Part model, mm, in its own coordinate system. A direction names the side the tool comes from. Give positions to 0.01 mm unless a question says otherwise; leave off trailing zeros. Write each loop counter-clockwise with the first axis right and the second up, starting at its lowest first coordinate (ties: lowest second). Pieces come first, ordered by that corner, then holes. Notation, with made-up numbers: M 62.5,-9.75 L 87.5,-9.75 A36 ccw 87.5,26.25 Z; hole C 64.5,41 d10. An arc over 180 degrees is marked long. Use a Markdown table: item, result. Add a question column.
from build123d import *

# Parameters (mm, degrees)
BOSS_EXTRUDE2_DEPTH = 34.29
CHAMFER1_SIZE       = 2.54
CHAMFER2_SIZE       = 2.54


with BuildPart() as part:
    # Sketch2 → Boss-Extrude2 (new body)
    with BuildSketch(Plane.XY):
        with BuildLine():
            Line((-29.230640855, 30.0736), (29.230640855, 30.0736))
            ThreePointArc((29.230640855, 30.0736), (33.347275907, 29.151687047), (36.677508311, 26.562061635))
            Line((36.677508311, 26.562061635), (49.972274675, 10.43878478))
            ThreePointArc((49.972274675, 10.43878478), (51.110407437, -8.880095747), (33.055391111, -15.846506335))
            Line((33.055391111, -15.846506335), (9.525, -9.525))
            Line((9.525, -9.525), (9.525, -4.1275))
            ThreePointArc((9.525, -4.1275), (10.268948776, -2.331448776), (12.065, -1.5875))
            Line((12.065, -1.5875), (28.178527264, -1.5875))
            ThreePointArc((28.178527264, -1.5875), (46.5836, 0), (28.178527264, 1.5875))
            Line((28.178527264, 1.5875), (-28.178527264, 1.5875))
            ThreePointArc((-28.178527264, 1.5875), (-46.5836, 0), (-28.178527264, -1.5875))
            Line((-28.178527264, -1.5875), (-12.065, -1.5875))
            ThreePointArc((-12.065, -1.5875), (-10.268948776, -2.331448776), (-9.525, -4.1275))
            Line((-9.525, -4.1275), (-9.525, -9.525))
            Line((-9.525, -9.525), (-33.055391111, -15.846506335))
            ThreePointArc((-33.055391111, -15.846506335), (-51.110407437, -8.880095747), (-49.972274675, 10.43878478))
            Line((-49.972274675, 10.43878478), (-36.677508311, 26.562061635))
            ThreePointArc((-36.677508311, 26.562061635), (-33.347275907, 29.151687047), (-29.230640855, 30.0736))
        make_face()
    extrude(amount=BOSS_EXTRUDE2_DEPTH)

    # Chamfer1
    chamfer1_edges = [part.edges().sort_by_distance(p)[0] for p in [
        (33.347275907, 29.151687047, 34.29),
        (0, 30.0736, 34.29),
        (-33.347275907, 29.151687047, 34.29),
        (-43.324891493, 18.500423208, 34.29),
        (-51.110407437, -8.880095747, 34.29),
        (-21.290195556, -12.685753168, 34.29),
        (-9.525, -6.82625, 34.29),
        (-10.268948776, -2.331448776, 34.29),
        (-20.121763632, -1.5875, 34.29),
        (-46.5836, 0, 34.29),
        (51.110407437, -8.880095747, 34.29),
        (0, 1.5875, 34.29),
        (46.5836, 0, 34.29),
        (20.121763632, -1.5875, 34.29),
        (10.268948776, -2.331448776, 34.29),
        (9.525, -6.82625, 34.29),
        (21.290195556, -12.685753168, 34.29),
        (43.324891493, 18.500423208, 34.29),
    ]]
    chamfer(chamfer1_edges, length=CHAMFER1_SIZE)

    # Chamfer2
    chamfer2_edges = [part.edges().sort_by_distance(p)[0] for p in [
        (21.290195556, -12.685753168, 0),
        (-21.290195556, -12.685753168, 0),
        (-51.110407437, -8.880095747, 0),
        (-43.324891493, 18.500423208, 0),
        (-33.347275907, 29.151687047, 0),
        (0, 30.0736, 0),
        (33.347275907, 29.151687047, 0),
        (43.324891493, 18.500423208, 0),
        (51.110407437, -8.880095747, 0),
    ]]
    chamfer(chamfer2_edges, length=CHAMFER2_SIZE)


solid = part.part
1. Cut at B-B (x = -25). Write the cut outline in (y, z), then the cut area to 3 significant figures.
2. Flat gauge pins, fed straight in: pin 1 (1 mm diameter, centred on x = -32, z = 29, fed in from -Y); pin 2 (3 mm diameter, centred on x = 11, z = 18, fed in from -Y); pin 3 (4.5 mm diameter, centred on y = -7, z = 13, fed in from +X); pin 4 (12 mm diameter, centred on x = -35.5, y = -3, fed in from -Z). Where does each tip first touch, or does it go through?
3. Cut at A-A (y = 0). Write the cut outline in (x, z), then the cut area to 3 significant figures.
4. Cut at C-C (z = 25.5). Write the cut outline in (x, y) (1 decimal), then the cut area to 3 significant figures.
5. Cut at D-D (x = 4). Write the cut outline in (y, z), then the cut area to 3 significant figures.
6. Mould opens along Y. For faces 1 (the flat face through (-42.42, 17.57, 33.04)), 2 (the conical face through (46.734, -0.392, 31.909)), 3 (the flat face through (-21.125, -12.642, 16.941)) say: released by +Y, released by -Y, zero draft, split by the parting line, or undercut.
7. Drill centre lines: probe 1 along X at (y, z) = (5, 2); probe 2 along X at (y, z) = (8.5, 4); probe 3 along X at (y, z) = (-6, 11) (3 decimals). Where is each one in solid material? Low to high. Write a range as [from, to].
8. Tool access for faces 4 (the flat face through (21.789, -11.486, 33.038)), 5 (the flat face through (-21.116, -11.342, 1.288)), 6 (the flat face through (9.525, -7, 16)), 7 (the cylindrical face through (-33.401, 29.126, 16.941)), 8 (the flat face through (20, -1.588, 16)): list every direction of +Z, -Z, +X, -X, +Y, -Y with a clear straight run to the whole face (end or side of a thin tool).
A:
| question | item | result |
|---|---|---|
| 1 | outline | M -13.68,2.54 L -11.05,0 L -1.59,0 L -1.59,31.75 L -4.13,34.29 L -11.05,34.29 L -13.68,31.75 Z; M 1.59,0 L 27.53,0 L 30.07,2.54 L 30.07,31.75 L 27.53,34.29 L 4.13,34.29 L 1.59,31.75 Z |
| 1 | area | 1,370 mm² |
| 2 | pin 1 | stops at y = -15.7 |
| 2 | pin 2 | stops at y = -10.32 |
| 2 | pin 3 | stops at x = 53.02 |
| 2 | pin 4 | stops at z = 0 |
| 3 | outline | M -53.72,2.54 L -51.18,0 L -46.58,0 L -46.58,31.75 L -49.12,34.29 L -51.18,34.29 L -53.72,31.75 Z; M 46.58,0 L 51.18,0 L 53.72,2.54 L 53.72,31.75 L 51.18,34.29 L 49.12,34.29 L 46.58,31.75 Z |
| 3 | area | 470 mm² |
| 4 | outline | M -50,10.4 A16.4 ccw -33.1,-15.8 L -9.5,-9.5 L -9.5,-4.1 A2.5 ccw -12.1,-1.6 L -28.2,-1.6 A9.3 cw long -28.2,1.6 L 28.2,1.6 A9.3 cw long 28.2,-1.6 L 12.1,-1.6 A2.5 ccw 9.5,-4.1 L 9.5,-9.5 L 33.1,-15.8 A16.4 ccw 50,10.4 L 36.7,26.6 A9.7 ccw 29.2,30.1 L -29.2,30.1 A9.7 ccw -36.7,26.6 Z |
| 4 | area | 3,200 mm² |
| 5 | outline | M 1.59,0 L 27.53,0 L 30.07,2.54 L 30.07,31.75 L 27.53,34.29 L 4.13,34.29 L 1.59,31.75 Z |
| 5 | area | 967 mm² |
| 6 | face 1 | released by +Y |
| 6 | face 2 | undercut |
| 6 | face 3 | released by -Y |
| 7 | probe 1 | x = [-52.37, -45.12], [-29.51, 29.51], [45.12, 52.37] |
| 7 | probe 2 | x = [-51.35, -41.01], [-33.61, 33.61], [41.01, 51.35] |
| 7 | probe 3 | x = [-52.585, -44.38], [-30.245, -9.525], [9.525, 30.245], [44.38, 52.585] |
| 8 | face 4 | +Z, -Y |
| 8 | face 5 | -Z, -Y |
| 8 | face 6 | +Z, -Z, -Y |
| 8 | face 7 | +Z, -Z, -X, +Y |
| 8 | face 8 | +Z, -Z |
